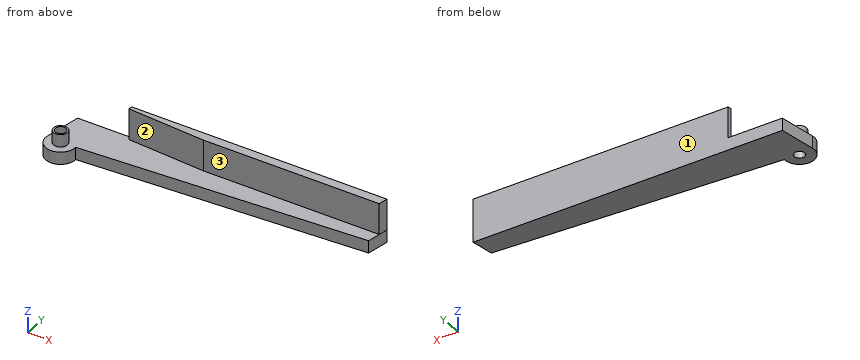
```python
from build123d import *

# Parameters (mm, degrees)
SKETCH001_R  = 1.7
PAD001_DEPTH = 4
PAD003_DEPTH = 10
SKETCH_R     = 2.25
SKETCH_R_2   = 1.7
PAD_DEPTH    = 4


with BuildPart() as part:
    # Sketch001 → Pad001 (new body)
    with BuildSketch(Plane.XY):
        with BuildLine():
            ThreePointArc((-4.677837, 0.824829), (-0.282136, -4.741614), (4.742642, 0.26429))
            Line((96.121215, 5.356476), (4.742642, 0.26429))
            Line((97.380811, 12.5), (96.121215, 5.356476))
            Line((-2.619189, 12.5), (97.380811, 12.5))
            Line((-4.677837, 0.824829), (-2.619189, 12.5))
        make_face()
        Circle(SKETCH001_R, mode=Mode.SUBTRACT)
    extrude(amount=-PAD001_DEPTH)

    # Sketch004 → Pad003 (join)
    with BuildSketch(Plane.XY):
        Polygon((14.896796, 12.5), (97.363709, 12.5), (96.825632, 9.5), (39.982536, 9.5), (14.684946, 11.318848), align=None)
    extrude(amount=PAD003_DEPTH)

    # Sketch → Pad (join)
    with BuildSketch(Plane.XY):
        Circle(SKETCH_R)
        Circle(SKETCH_R_2, mode=Mode.SUBTRACT)
    extrude(amount=PAD_DEPTH)


solid = part.part
```
Could you check a few things on this model? Use its own coordinates, in mm. Face numbers are marked on the shaded views. A direction names the side the tool comes from. Give positions to 0.01 mm unless a question says otherwise; leave off trailing zeros. Loops run counter-clockwise (first coordinate to the right, second up) from the corner with the lowest first, then second, coordinate; pieces in that order, holes last. Notation, with made-up numbers: (-30, -26.75) - (23, -26.75) arc R9 cw to (23, -12.75) - close; hole circle Ø11 at (-40, 43). An arc over 180 degrees is marked (long way). Answer in a Markdown table with one row per item. Add a question column.
Q1. If we section it at A-A (z = 1.25): List the corners of the cut face in (x, y) for me.
Q2. Which directions (+Z, -Z, +X, -X, +Y, -Y) give clear straight access to the entire face, cutting with the end or side of a thin tool? Please do the marked faces 1, 2 and 3.
Q3. If we section it at B-B (x = 0): List the corners of the cut face in (y, z) for me.
Q4. If we section it at D-D (x = 55): List the corners of the cut face in (y, z) for me, plus the area to 3 significant figures.
Q5. For pin 1 (4.5 mm diameter, centred on x = 0, y = 0, fed in from -Z); pin 2 (4 mm diameter, centred on y = 7, z = 7, fed in from -X) (3 decimals); pin 3 (3 mm diameter, centred on x = 71.5, z = 3, fed in from -Y); pin 4 (2 mm diameter, centred on x = -1, y = 0, fed in from +Z), each with a flat end and sliding along its axis, tell me the tip position at first contact or that it passes through.
Q6. Please list where these lines run through material, in increasing order: L1, parallel to Y at x = 0, z = -1; L2, parallel to Y at x = 0, z = 0.5; L3, parallel to Z at x = 38, y = 7.75. Write a range as from..to.
Q7. If we section it at C-C (z = 5.5): List the corners of the cut face in (x, y) for me.
The answers:
| question | item | result |
|---|---|---|
| 1 | outline | circle Ø4.5 at (0, 0); (14.68, 11.32) - (39.98, 9.5) - (96.83, 9.5) - (97.36, 12.5) - (14.9, 12.5) - close; hole circle Ø3.4 at (0, 0) |
| 2 | face 1 | +Z, -Z, +X, -X, +Y |
| 2 | face 2 | +Z, -X, -Y |
| 2 | face 3 | +Z, +X, -X, -Y |
| 3 | outline | (-4.75, -4) - (-1.7, -4) - (-1.7, 4) - (-2.25, 4) - (-2.25, 0) - (-4.75, 0) - close; (1.7, -4) - (12.5, -4) - (12.5, 0) - (2.25, 0) - (2.25, 4) - (1.7, 4) - close |
| 4 | outline | (3.06, -4) - (12.5, -4) - (12.5, 10) - (9.5, 10) - (9.5, 0) - (3.06, 0) - close |
| 4 | area | 67.7 mm^2 |
| 5 | pin 1 | stops at z = -4 |
| 5 | pin 2 | passes through |
| 5 | pin 3 | stops at y = 9.5 |
| 5 | pin 4 | stops at z = 4 |
| 6 | L1 | y = -4.75..-1.7, 1.7..12.5 |
| 6 | L2 | y = -2.25..-1.7, 1.7..2.25 |
| 6 | L3 | z = -4..0 |
| 7 | outline | (14.68, 11.32) - (39.98, 9.5) - (96.83, 9.5) - (97.36, 12.5) - (14.9, 12.5) - close |
